Work out the finished part from the listing and answer in its coordinate system (mm). A direction names the side the tool comes from. Round coordinates to 2 decimals unless told otherwise and drop trailing zeros. Loops run counter-clockwise (first coordinate to the right, second up) from the corner with the lowest first, then second, coordinate; pieces in that order, holes last. Notation, with made-up numbers: (32, 60.5) -> (56, 60.5) arc R29 cw to (56, 93.5) -> close; hole circle Ø8 at (40.5, 68.25). An arc over 180 degrees is marked (long way). Write item = value, one per line. Start each with the question number.
Autodesk Inventor part; units mm, degrees
ref_plane "YZ Plane" through (0, 0, 0) normal (1, 0, 0) x (0, 1, 0)
ref_plane "XZ Plane" through (0, 0, 0) normal (0, 1, 0) x (-1, 0, 0)
ref_plane "XY Plane" through (0, 0, 0) normal (0, 0, 1) x (1, 0, 0)
sketch "スケッチ1" plane through (0, 0, 0) normal (0, 0, 1) x (1, 0, 0)
  circle A0 centre (0, 0) radius 3
  circle A1 centre (0, 0) radius 1.5
  dimension "d0" = 6
  dimension "d1" = 3
extrude "押し出し1" add sketch "スケッチ1" along normal blind 30
fillet "フィレット1" radius 0.3 2 edges at (-3, 0, 30) (-3, 0, 0)
thread "ねじ1"
extrude "押し出し2" add sketch "スケッチ1" along normal blind 24 contours A1
extrude "押し出し3" cut sketch "スケッチ1" along normal blind 6 contours A1
thread "ねじ2"
properties part number "スペーサーM3L30アルミ" material "アルミニウム 2014-T4"
Item 1: A tool of negligible diameter and unlimited length cuts with its end or side. For faces 1 (the flat face through (0, 0, 24)), 2 (the flat face through (1.2, -1.2, 0)), from which of +Z, -Z, +X, -X, +Y, -Y can it reach the whole face along a straight path? Write none if from no direction.
Item 2: Section B-B (y = 0) is taken. Determine the outline of the cut face in (x, z).
Item 3: Section A-A (z = 2.5) is taken. Determine the outline of the cut face in (x, y).
Item 4: Section D-D (z = 13.5) is taken. Determine the outline of the cut face in (x, y), then the cut area to 3 significant figures.
Item 5: The mould has two halves that part along Y. Classify faces 3 (the cylindrical face through (-1.5, -0.07, 2.96)), 4 (the cylindrical face through (-3, 0, 15)), 5 (the flat face through (1.2, -1.2, 30)), 6 (the flat face through (0, 0, 6)): pulls with the +Y half, pulls with the -Y half, needs draft (parallel to the pull), parting line crosses it, or undercut.
Item 6: Find the intervals of material crossed by line 1 along Y through (x, z) = (0, 28.05); line 2 along Z through (x, y) = (1, -1); line 3 along Y through (x, z) = (-0.75, 14.5), in increasing order. Write a range as [from, to].
Item 7: Flat-ended cylindrical pins translate along their axes: pin 1 (3 mm diameter, centred on y = -2.5, z = 5, fed in from +X); pin 2 (1.5 mm diameter, centred on x = 0, y = 0.5, fed in from -Z); pin 3 (2 mm diameter, centred on x = -1.5, z = 4, fed in from -Y). Find the tip coordinate at first contact, or state that the pin passes through.
Worked answers:
q1.face_1 = +Z
q1.face_2 = -Z, +X, -X, +Y, -Y
q2.outline = (-3, 0.3) arc R0.3 ccw to (-2.7, 0) -> (-1.5, 0) -> (-1.5, 6) -> (1.5, 6) -> (1.5, 0) -> (2.7, 0) arc R0.3 ccw to (3, 0.3) -> (3, 29.7) arc R0.3 ccw to (2.7, 30) -> (1.5, 30) -> (1.5, 24) -> (-1.5, 24) -> (-1.5, 30) -> (-2.7, 30) arc R0.3 ccw to (-3, 29.7) -> close
q3.outline = circle Ø6 at (0, 0); hole circle Ø3 at (0, 0)
q4.outline = circle Ø6 at (0, 0)
q4.area = 28.3 mm2
q5.face_3 = undercut
q5.face_4 = parting line crosses it
q5.face_5 = needs draft
q5.face_6 = undercut
q6.line_1 = [-3, -1.5], [1.5, 3]
q6.line_2 = [6, 24]
q6.line_3 = [-2.9, 2.9]
q7.pin_1 = 2.83
q7.pin_2 = 6
q7.pin_3 = -2.96
